Design review of the part built by this model. Coordinates are the model's own, in mm. A direction names the side the tool comes from. Give positions to 0.01 mm unless a question says otherwise; leave off trailing zeros. Write each loop counter-clockwise with the first axis right and the second up, starting at its lowest first coordinate (ties: lowest second). Pieces come first, ordered by that corner, then holes. Notation, with made-up numbers: (76.25, 35) -> (123.25, 35) arc R26 ccw to (123.25, 49) -> close; hole circle Ø2 at (19, 88.25). An arc over 180 degrees is marked (long way). Put each result on its own line as item: value. Start each with the question number.
from build123d import *

# Parameters (mm, degrees)
F0_W     = 30
F0_H     = 20
F1_DEPTH = 10
F2_W     = 5
F2_H     = 20
F3_DEPTH = 5
F4_R     = 2.5
F5_DEPTH = 10.001
F7_DEPTH = 10.001
F8_W     = 10
F8_H     = 5
F9_DEPTH = 30.001


with BuildPart() as f1:
    # F0 (on Top) → F1 (new body)
    with BuildSketch(Plane.XY):
        with Locations((4.2107195362, -27.6951151714)):
            Rectangle(F0_W, F0_H)
    extrude(amount=F1_DEPTH)

    # F2 (on face) → F3 (join)
    with BuildSketch(Plane.XY.offset(10)):
        with Locations((-8.2892804638, -27.6951151714)):
            Rectangle(F2_W, F2_H)
        with Locations((16.7107195362, -27.6951151714)):
            Rectangle(F2_W, F2_H)
    extrude(amount=F3_DEPTH)

    # F4 (on face) → F5 (cut, through all)
    with BuildSketch(Plane.XY.offset(10)):
        with Locations((-0.7892804638, -27.6951151714)):
            Circle(F4_R)
    extrude(amount=-F5_DEPTH, mode=Mode.SUBTRACT)

    # F6 (on face) → F7 (cut, through all)
    with BuildSketch(Plane.XY.offset(10)):
        with BuildLine():
            ThreePointArc((9.2107195362, -25.1951151714), (6.7107195362, -27.6951151714), (9.2107195362, -30.1951151714))
            Line((9.2107195362, -30.1951151714), (9.2107195362, -25.1951151714))
        make_face()
        with BuildLine():
            Line((9.2107195362, -25.1951151714), (9.2107195362, -30.1951151714))
            ThreePointArc((9.2107195362, -30.1951151714), (10.9784864892, -29.4628821243), (11.7107195362, -27.6951151714))
            ThreePointArc((11.7107195362, -27.6951151714), (10.9784864892, -25.9273482184), (9.2107195362, -25.1951151714))
        make_face()
    extrude(amount=-F7_DEPTH, mode=Mode.SUBTRACT)

    # F8 (on face) → F9 (cut, through all)
    with BuildSketch(Plane.YZ.offset(19.2107195362)):
        with Locations((-27.6951151714, 2.5)):
            Rectangle(F8_W, F8_H)
    extrude(amount=-F9_DEPTH, mode=Mode.SUBTRACT)


solid = f1.part
Q1. Take a section at D-D on z = 5.5. Give the boundary of the cut face in (x, y).
Q2. For pin 1 (5 mm diameter, centred on x = 4, y = -29, fed in from -Z); pin 2 (6 mm diameter, centred on x = -5.5, z = 12, fed in from +Y); pin 3 (2 mm diameter, centred on x = 1, y = -29.5, fed in from +Z), all flat-tipped, find the tip position at first contact; note any pin that passes through.
Q3. Machinability: for faces 1 (the face through (-5.789, -28, 12)), 2 (the face through (4, -32.695, 2)), 3 (the face through (17, -28, 15)), which of the approach directions +Z, -Z, +X, -X, +Y, -Y give a long, thin tool a straight path to every point of the face, cutting with its end or side? Answer none if there is none.
Q4. Take a section at A-A on z = 12.75. Give the boundary of the cut face in (x, y), then the cut area to 3 significant figures.
Q5. Take a section at B-B on y = -26.25. Give the boundary of the cut face in (x, z).
Q6. Mouldability with a two-part tool opening along Y and no side actions: class faces 4 (the face through (-10.789, -28, 9)), 5 (the face through (4, -37.695, 6)), 6 (the face through (4, -17.695, 6)), 7 (the face through (4, -22.695, 2)) as +Y half, -Y half, draft (parallel to the pull), parting line (faces both ways), or undercut.
Q7. To check wall thickness, follow probe 1 along Y at (x, z) = (5.75, 3.5); probe 2 along X at (y, z) = (-32.75, 10.5); probe 3 along X at (y, z) = (-26, 6.5). State the ranges of each line that lie inside material, in increasing order. Write a range as from..to.
Q8. Take a section at C-C on x = 7.5. Give the boundary of the cut face in (y, z).
Result:
1. outline: (-10.79, -37.7) -> (19.21, -37.7) -> (19.21, -17.7) -> (-10.79, -17.7) -> close; hole circle Ø5 at (-0.79, -27.7); hole circle Ø5 at (9.21, -27.7)
2. pin 1: stops at z = 5
2. pin 2: stops at y = -17.7
2. pin 3: stops at z = 10
3. face 1: +Z, +Y, -Y
3. face 2: -Z, +X, -X
3. face 3: +Z, +X, -X, +Y, -Y
4. outline: (-10.79, -37.7) -> (-5.79, -37.7) -> (-5.79, -17.7) -> (-10.79, -17.7) -> close; (14.21, -37.7) -> (19.21, -37.7) -> (19.21, -17.7) -> (14.21, -17.7) -> close
4. area: 200 mm^2
5. outline: (-10.79, 5) -> (-2.83, 5) -> (-2.83, 10) -> (-5.79, 10) -> (-5.79, 15) -> (-10.79, 15) -> close; (1.25, 5) -> (7.17, 5) -> (7.17, 10) -> (1.25, 10) -> close; (11.25, 5) -> (19.21, 5) -> (19.21, 15) -> (14.21, 15) -> (14.21, 10) -> (11.25, 10) -> close
6. face 4: draft
6. face 5: -Y half
6. face 6: +Y half
6. face 7: undercut
7. probe 1: y = -37.7..-32.7, -22.7..-17.7
7. probe 2: x = -10.79..-5.79, 14.21..19.21
7. probe 3: x = -10.79..-2.63, 1.05..7.37, 11.05..19.21
8. outline: (-37.7, 0) -> (-32.7, 0) -> (-32.7, 5) -> (-29.52, 5) -> (-29.52, 10) -> (-37.7, 10) -> close; (-25.87, 5) -> (-22.7, 5) -> (-22.7, 0) -> (-17.7, 0) -> (-17.7, 10) -> (-25.87, 10) -> close
